Autodesk Inventor part; units mm, degrees
ref_plane "YZ Plane" through (0, 0, 0) normal (1, 0, 0) x (0, 1, 0)
ref_plane "XZ Plane" through (0, 0, 0) normal (0, 1, 0) x (-1, 0, 0)
ref_plane "XY Plane" through (0, 0, 0) normal (0, 0, 1) x (1, 0, 0)
sketch "Sketch1" plane through (0, 0, 0) normal (0, 0, 1) x (1, 0, 0)
  arc A0 (-3.5858, 30.4056) -> (-7.1213, 28.9411) centre (-3.5858, 25.4056) ccw
  line L0 (-7.1213, 28.9411) -> (-28.9411, 7.1213)
  arc A1 (-28.9411, 7.1213) -> (-30.4056, 3.5858) centre (-25.4056, 3.5858) ccw
  line L1 (-30.4056, 3.5858) -> (-30.4056, -3.5858)
  arc A2 (-30.4056, -3.5858) -> (-28.9411, -7.1213) centre (-25.4056, -3.5858) ccw
  line L2 (-28.9411, -7.1213) -> (-7.1213, -28.9411)
  arc A3 (-7.1213, -28.9411) -> (-3.5858, -30.4056) centre (-3.5858, -25.4056) ccw
  line L3 (-3.5858, -30.4056) -> (3.5858, -30.4056)
  arc A4 (3.5858, -30.4056) -> (7.1213, -28.9411) centre (3.5858, -25.4056) ccw
  line L4 (7.1213, -28.9411) -> (22.1833, -13.8792)
  arc A5 (16, -5.7446) -> (22.1833, -13.8792) centre (32, 0) ccw
  arc A6 (16, 5.7446) -> (16, -5.7446) centre (0, 0) ccw
  arc A7 (22.1833, 13.8792) -> (16, 5.7446) centre (32, 0) ccw
  line L5 (22.1833, 13.8792) -> (7.1213, 28.9411)
  arc A8 (7.1213, 28.9411) -> (3.5858, 30.4056) centre (3.5858, 25.4056) ccw
  line L6 (3.5858, 30.4056) -> (-3.5858, 30.4056)
  circle A9 centre (-8.1317, 22.2739) radius 1.5
  circle A10 centre (-22.2739, 8.1317) radius 1.5
  circle A11 centre (8.1317, -22.2739) radius 1.5
  circle A12 centre (-8.1317, -22.2739) radius 1.5
  circle A13 centre (8.1317, 22.2739) radius 1.5
  circle A14 centre (-22.2739, -8.1317) radius 1.5
  point P0 (0, 0)
extrude "Extrusion1" add sketch "Sketch1" along normal blind 3
fillet "Fillet1" radius 1 4 edges at (16, 5.7446, 1.5) (22.1833, 13.8792, 1.5) (16, -5.7446, 1.5) (22.1833, -13.8792, 1.5)
properties part number "VAM_housing_top"
Geometry: final body of the model. Coordinates: model frame, mm. Round coordinates to 2 decimals unless told otherwise and drop trailing zeros. Order: outer loops, then holes, each group sorted by start corner. A loop starts at its lowest first (then second) coordinate and runs counter-clockwise, first axis right, second up. Notation, with made-up numbers: (-7.75, 82.5) -> (44.25, 82.5) arc R27 ccw to (44.25, 120.5) -> close; hole circle Ø10 at (50.25, 7). An arc over 180 degrees is marked (long way). Put each result on its own line as item: value. Start each with the question number.
Q1. Pull-direction query (X, two-part tool) for faces 1 (the cylindrical face through (18.78, 10.69, 1.48)), 2 (the flat face through (0, -30.406, 1)), 3 (the cylindrical face through (9.517, 22.848, 1.479)); classes: +X half, -X half, draft (parallel to the pull), parting line (faces both ways), or undercut.
Q2. Line query: probe 1 along Y at (x, z) = (-21, 0.7); probe 2 along X at (y, z) = (9, 1.95); probe 3 along X at (y, z) = (-11, 1.3). Output: solid intervals per line, ascending.
Q3. Section A-A on x = 0. Return the cut outline in (y, z).
Q4. Section C-C on y = 0. Return the cut outline in (x, z).
Q5. Section D-D on z = 0.8. Give the number of separate pieces and of enclosed holes in the cut face, and give its area (3 significant figures).
Q6. First-contact query: pin 1 (3.5 mm diameter, centred on x = -22.27, y = -8.13, fed in from -Z). Flat tip, straight axial feed; report the tip coordinate or a pass-through.
Q7. Section B-B on x = 13.5. Return the cut outline in (y, z), and give its area (3 significant figures).
Ans:
1. face 1: +X half
1. face 2: draft
1. face 3: undercut
2. probe 1: y = -15.06 to -8.92, -7.34 to 7.34, 8.92 to 15.06
2. probe 2: x = -27.06 to -23.5, -21.05 to -14.42, 14.42 to 17.58
2. probe 3: x = -25.06 to -12.96, 12.96 to 19.04
3. outline: (-30.41, 0) -> (-17, 0) -> (-17, 3) -> (-30.41, 3) -> close; (17, 0) -> (30.41, 0) -> (30.41, 3) -> (17, 3) -> close
4. outline: (-30.41, 0) -> (-17, 0) -> (-17, 3) -> (-30.41, 3) -> close
5. separate pieces: 1
5. enclosed holes: 6
5. area: 1,230 mm2
6. pin 1: stops at z = 0
7. outline: (-22.56, 0) -> (-10.33, 0) -> (-10.33, 3) -> (-22.56, 3) -> close; (10.33, 0) -> (22.56, 0) -> (22.56, 3) -> (10.33, 3) -> close
7. area: 73.4 mm2
